Model file for the job. Use its own axes, mm. Coordinates: 2 decimals unless noted, no trailing zeros. Loops run counter-clockwise (first coordinate to the right, second up) from the corner with the lowest first, then second, coordinate; pieces in that order, holes last.
from build123d import *

# Parameters (mm, degrees)
SKETCH_1_W               = 100
SKETCH_1_H               = 43
EXTRUDE_1_DEPTH          = 8
SKETCH_2_R               = 1.3
CUT_EXTRUDE_1_DEPTH      = 8
PATTERN_LINEAR_1_COUNT   = 3
PATTERN_LINEAR_1_PITCH   = 42
MIRROR_1_COPY_1_SKETCH_R = 1.3
MIRROR_1_COPY_1_DEPTH    = 8
MIRROR_1_COPY_2_SKETCH_R = 1.3
MIRROR_1_COPY_2_DEPTH    = 8
CHAMFER_1_SIZE           = 0.2


with BuildPart() as part:
    # 草圖1 → 填料-伸長1 (new body)
    with BuildSketch(Plane.XY):
        Rectangle(SKETCH_1_W, SKETCH_1_H)
    extrude(amount=EXTRUDE_1_DEPTH)

    # 草圖2 → 除料-伸長1 (cut)
    with BuildSketch(Plane(origin=(0, 21.5, 0), x_dir=(1, 0, 0), z_dir=(0, 1, 0))):
        with Locations(Location((-42, -4, 0), (0, 0, 270))):
            Circle(SKETCH_2_R)
    cut_extrude_1 = extrude(amount=-CUT_EXTRUDE_1_DEPTH, mode=Mode.SUBTRACT)

    # 直線複製排列1: 除料-伸長1 ×3
    with Locations(*[(i * PATTERN_LINEAR_1_PITCH, 0, 0) for i in range(1, PATTERN_LINEAR_1_COUNT)]):
        add(cut_extrude_1, mode=Mode.SUBTRACT)

    # 鏡射1: 除料-伸長1 across plane
    add(cut_extrude_1.mirror(Plane.ZX), mode=Mode.SUBTRACT)

    # 鏡射1 copy 1 sketch → 鏡射1 copy 1 (cut)
    with BuildSketch(Plane(origin=(42, -21.5, 0), x_dir=(1, 0, 0), z_dir=(0, -1, 0))):
        with Locations((-42, 4)):
            Circle(MIRROR_1_COPY_1_SKETCH_R)
    extrude(amount=-MIRROR_1_COPY_1_DEPTH, mode=Mode.SUBTRACT)

    # 鏡射1 copy 2 sketch → 鏡射1 copy 2 (cut)
    with BuildSketch(Plane(origin=(84, -21.5, 0), x_dir=(1, 0, 0), z_dir=(0, -1, 0))):
        with Locations((-42, 4)):
            Circle(MIRROR_1_COPY_2_SKETCH_R)
    extrude(amount=-MIRROR_1_COPY_2_DEPTH, mode=Mode.SUBTRACT)

    # 導角1
    chamfer_1_edges = [part.edges().sort_by_distance(p)[0] for p in [
        (-42, 21.5, 2.7),
        (0, 21.5, 2.7),
        (42, 21.5, 2.7),
        (-42, -21.5, 2.7),
        (-1.3, -21.5, 4),
        (40.7, -21.5, 4),
    ]]
    chamfer(chamfer_1_edges, length=CHAMFER_1_SIZE)


solid = part.part
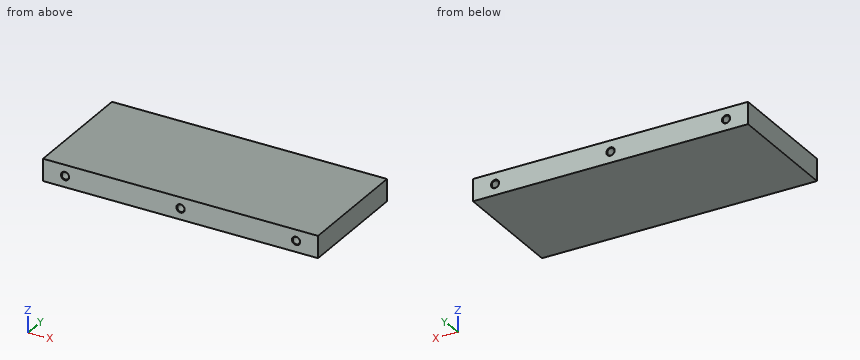
Q1. Flat gauge pins, fed straight in: P1, Ø2, axis at x = 0, z = 4, coming from the +Y side; P2, Ø1.6, axis at x = -42, z = 4, coming from the -Y side. Where does each tip first touch, or does it go through?
Answers:
P1: stops at y = 13.5
P2: stops at y = -13.5
Q2. Slice it at A-A (y = 18). List the corners of the cut face in (x, z).
Answers:
outline: (-50, 0) - (50, 0) - (50, 8) - (-50, 8) - close; hole circle Ø2.6 at (-42, 4); hole circle Ø2.6 at (0, 4); hole circle Ø2.6 at (42, 4)
Q3. Drill centre lines: line 1 (X direction, y = 17.5, z = 4); line 2 (Z direction, x = 42, y = -18). Where is each one in solid material? Low to high.
Answers:
line 1: x = -50 to -43.3, -40.7 to -1.3, 1.3 to 40.7, 43.3 to 50
line 2: z = 0 to 2.7, 5.3 to 8
Q4. Slice it at B-B (x = 42). List the corners of the cut face in (y, z), and give its area (3 significant figures).
Answers:
outline: (-21.5, 0) - (21.5, 0) - (21.5, 2.5) - (21.3, 2.7) - (13.5, 2.7) - (13.5, 5.3) - (21.3, 5.3) - (21.5, 5.5) - (21.5, 8) - (-21.5, 8) - (-21.5, 5.5) - (-21.3, 5.3) - (-13.5, 5.3) - (-13.5, 2.7) - (-21.3, 2.7) - (-21.5, 2.5) - close
area: 302 mm2
